Could you check a few things on this drawing? It's one solid part, dimensions in mm from its lowest x, y, z. Round coordinates to 2 decimals unless told otherwise and drop trailing zeros. Order: outer loops, then holes, each group sorted by start corner. A loop starts at its lowest first (then second) coordinate and runs counter-clockwise, first axis right, second up. Notation, with made-up numbers: (-28.5, 77.25) -> (21.5, 77.25) arc R34 cw to (21.5, 115.25) -> close; hole circle Ø5 at (-5.75, 86). An arc over 180 degrees is marked (long way). Use a Markdown table: item, result. Add a question column.
(1) I want a section at D-D, the plane x = 44.5. Please give me the cut outline in (y, z).
(2) I'm going to push flat-ended pins straight in: P1, Ø1.5, axis at x = 64.5, y = 1, coming from the +Z side; P2, Ø2, axis at x = 34.5, z = 15.5, coming from the -Y side; P3, Ø1.5, axis at x = 21.5, y = 1.5, coming from the -Z side; P4, Ø0.9, axis at x = 64, y = 2, coming from the -Z side. Where does each tip first touch, or does it pass through?
(3) If I drill on probe 1 along X at (y, z) = (0.6, 13); probe 2 along X at (y, z) = (2.6, 3.25); probe 3 along Z at (x, y) = (12.05, 1.1) (1 decimal), over which ranges is the centre line in solid material (lowest first)?
(4) I want a section at A-A, the plane x = 12.05. Please give me the cut outline in (y, z).
(5) I want a section at B-B, the plane y = 2. Please give me the cut outline in (x, z).
(6) I want a section at C-C, the plane z = 13. Please give me the cut outline in (x, y), then the cut area to 3 significant figures.
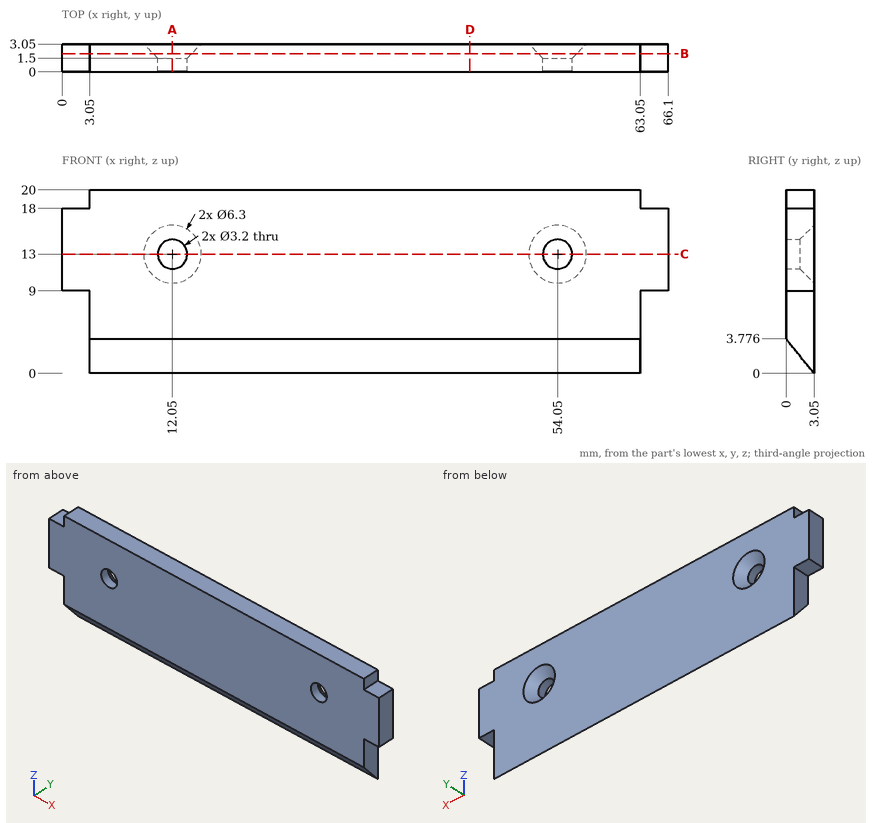
Taken from the geometry:
| question | item | result |
|---|---|---|
| 1 | outline | (0, 3.78) -> (3.05, 0) -> (3.05, 20) -> (0, 20) -> close |
| 2 | P1 | stops at z = 18 |
| 2 | P2 | stops at y = 0 |
| 2 | P3 | stops at z = 0.99 |
| 2 | P4 | stops at z = 9 |
| 3 | probe 1 | x = 0 to 10.45, 13.65 to 52.45, 55.65 to 66.1 |
| 3 | probe 2 | x = 3.05 to 63.05 |
| 3 | probe 3 | z = 2.4 to 11.4, 14.6 to 20 |
| 4 | outline | (0, 3.78) -> (3.05, 0) -> (3.05, 9.85) -> (1.5, 11.4) -> (0, 11.4) -> close; (0, 14.6) -> (1.5, 14.6) -> (3.05, 16.15) -> (3.05, 20) -> (0, 20) -> close |
| 5 | outline | (0, 9) -> (3.05, 9) -> (3.05, 1.3) -> (63.05, 1.3) -> (63.05, 9) -> (66.1, 9) -> (66.1, 18) -> (63.05, 18) -> (63.05, 20) -> (3.05, 20) -> (3.05, 18) -> (0, 18) -> close; hole circle Ø4.2 at (12.05, 13); hole circle Ø4.2 at (54.05, 13) |
| 6 | outline | (0, 0) -> (10.45, 0) -> (10.45, 1.5) -> (8.9, 3.05) -> (0, 3.05) -> close; (13.65, 0) -> (52.45, 0) -> (52.45, 1.5) -> (50.9, 3.05) -> (15.2, 3.05) -> (13.65, 1.5) -> close; (55.65, 0) -> (66.1, 0) -> (66.1, 3.05) -> (57.2, 3.05) -> (55.65, 1.5) -> close |
| 6 | area | 177 mm2 |
